```python
from build123d import *

# Parameters (mm, degrees)
SALIENTE_EXTRUIR1_DEPTH = 6
REDONDEO1_R             = 0.8


with BuildPart() as part:
    # Croquis1 → Saliente-Extruir1 (new body)
    with BuildSketch(Plane.XY):
        with BuildLine():
            Line((0, 6.85), (150, 6.85))
            Line((150, 6.85), (150, 2.85))
            Line((150, 2.85), (156, 2.85))
            Line((156, 2.85), (156, 6.85))
            Line((156, 6.85), (384.75, 6.85))
            ThreePointArc((384.75, 6.85), (391.6, 0), (384.75, -6.85))
            Line((384.75, -6.85), (0, -6.85))
            ThreePointArc((0, -6.85), (-6.85, 0), (0, 6.85))
        make_face()
        with BuildLine():
            Line((0, 5.5), (148.65, 5.5))
            Line((148.65, 5.5), (148.65, 1.5))
            Line((148.65, 1.5), (157.35, 1.5))
            Line((157.35, 1.5), (157.35, 5.5))
            Line((157.35, 5.5), (384.75, 5.5))
            ThreePointArc((384.75, 5.5), (390.25, 0), (384.75, -5.5))
            Line((384.75, -5.5), (0, -5.5))
            ThreePointArc((0, -5.5), (-5.5, 0), (0, 5.5))
        make_face(mode=Mode.SUBTRACT)
    extrude(amount=SALIENTE_EXTRUIR1_DEPTH)

    # Redondeo1
    redondeo1_edges = [part.edges().sort_by_distance(p)[0] for p in [
        (150, 6.85, 3),
        (150, 2.85, 3),
        (156, 2.85, 3),
        (156, 6.85, 3),
        (157.35, 5.5, 3),
        (157.35, 1.5, 3),
        (148.65, 1.5, 3),
        (148.65, 5.5, 3),
    ]]
    fillet(redondeo1_edges, radius=REDONDEO1_R)


solid = part.part
```
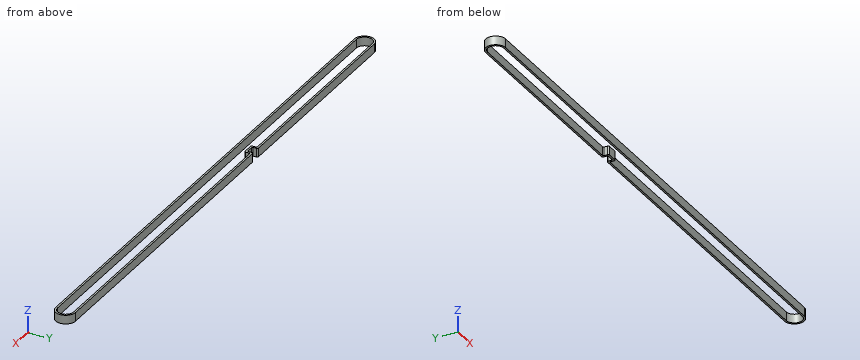
Could you check a few things on this model? Use its own coordinates, in mm. Round coordinates to 2 decimals unless told otherwise and drop trailing zeros. Order: outer loops, then holes, each group sorted by start corner. A loop starts at its lowest first (then second) coordinate and runs counter-clockwise, first axis right, second up. Notation, with made-up numbers: (17.5, 9.5) -> (38.5, 9.5) arc R25 ccw to (38.5, 24.5) -> close; hole circle Ø5 at (3, 19). An arc over 180 degrees is marked (long way). One line per question, with ' | ' between items.
Q1. If we section it at B-B on x = 338: Write out the boundary of the cut face in (y, z).
Computed values:
outline: (-6.85, 0) -> (-5.5, 0) -> (-5.5, 6) -> (-6.85, 6) -> close; (5.5, 0) -> (6.85, 0) -> (6.85, 6) -> (5.5, 6) -> close
Q2. If we section it at C-C on y = -2.25: Write out the boundary of the cut face in (x, z).
Computed values:
outline: (-6.47, 0) -> (-5.02, 0) -> (-5.02, 6) -> (-6.47, 6) -> close; (389.77, 0) -> (391.22, 0) -> (391.22, 6) -> (389.77, 6) -> close
Q3. I'm going to push flat-ended pins straight in: pin 1 (8 mm diameter, centred on x = 299, y = 5, fed in from +Z); pin 2 (1 mm diameter, centred on y = 5, z = 4.5, fed in from +X); pin 3 (5 mm diameter, centred on x = 243, y = 1, fed in from +Z); pin 4 (1.2 mm diameter, centred on y = 4.5, z = 4.5, fed in from +X). Where does each tip first touch, or does it pass through?
Computed values:
pin 1: z = 6 | pin 2: x = 389.91 | pin 3: through | pin 4: x = 390.38
Q4. If I drill on line 1 (Y direction, x = 29, z = 0.8); line 2 (X direction, y = 5, z = 5.55), over which ranges is the centre line in solid material (lowest first)? Write a range as from..to.
Computed values:
line 1: -6.85..-5.5, 5.5..6.85 | line 2: -4.68..-2.29, 148.59..150, 156..157.41, 387.04..389.43
Q5. If we section it at A-A on z = 1.6: Write out the boundary of the cut face in (x, y), plus the area to 3 significant figures.
Computed values:
outline: (0, -6.85) -> (384.75, -6.85) arc R6.85 ccw to (384.75, 6.85) -> (156.8, 6.85) arc R0.8 ccw to (156, 6.05) -> (156, 3.65) arc R0.8 cw to (155.2, 2.85) -> (150.8, 2.85) arc R0.8 cw to (150, 3.65) -> (150, 6.05) arc R0.8 ccw to (149.2, 6.85) -> (0, 6.85) arc R6.85 ccw to start; hole (0, -5.5) -> (384.75, -5.5) arc R5.5 ccw to (384.75, 5.5) -> (158.15, 5.5) arc R0.8 ccw to (157.35, 4.7) -> (157.35, 2.3) arc R0.8 cw to (156.55, 1.5) -> (149.45, 1.5) arc R0.8 cw to (148.65, 2.3) -> (148.65, 4.7) arc R0.8 ccw to (147.85, 5.5) -> (0, 5.5) arc R5.5 ccw to start | area: 1,100 mm²
